```python
from build123d import *

# Parameters (mm, degrees)
F1_DEPTH = 5.842
F3_D     = 6.35
F4_SIZE  = 0.508


with BuildPart() as f1:
    # F0 (on Front) → F1 (new body)
    with BuildSketch(Plane.XZ):
        with BuildLine():
            ThreePointArc((-9.5238039492, 50.4641557941), (-0.0754731213, 40.7885133075), (9.525, 50.3132142901))
            ThreePointArc((9.525, 50.3132142901), (9.5247764361, 50.3784740944), (9.524105755, 50.4437308352))
            ThreePointArc((9.524105755, 50.4437308352), (0.0102135943, 59.8382088142), (-9.5238039492, 50.4641557941))
        make_face()
        with BuildLine():
            ThreePointArc((9.524105755, 50.4437308352), (9.5247764361, 50.3784740944), (9.525, 50.3132142901))
            ThreePointArc((9.525, 50.3132142901), (-0.0754731213, 40.7885133075), (-9.5238039492, 50.4641557941))
            Line((-9.5238039492, 50.4641557941), (-15.7481848278, 1.515787542))
            ThreePointArc((-15.7481848278, 1.515787542), (-0.7382390734, 15.3710397423), (15.4940214613, 2.9702251313))
            Line((15.4940214613, 2.9702251313), (9.524105755, 50.4437308352))
        make_face()
        with BuildLine():
            Line((15.8675349274, 0), (15.4940214613, 2.9702251313))
            ThreePointArc((15.4940214613, 2.9702251313), (-0.7382390734, 15.3710397423), (-15.7481848278, 1.515787542))
            ThreePointArc((-15.7481848278, 1.515787542), (-15.8446680698, 0.4940908149), (-15.8749364489, -0.5317049948))
            Line((-15.8749364489, -0.5317049948), (-15.404151012, -4.3244616471))
            ThreePointArc((-15.404151012, -4.3244616471), (-0.1436036046, -16.3611361849), (15.332202426, -4.602510891))
            Line((15.332202426, -4.602510891), (15.8675349274, 0))
        make_face()
        with BuildLine():
            ThreePointArc((15.8675349274, 0), (15.7509480386, 1.4939366044), (15.4940214613, 2.9702251313))
            Line((15.4940214613, 2.9702251313), (15.8675349274, 0))
        make_face()
        with BuildLine():
            ThreePointArc((-15.8749364489, -0.5317049948), (-15.8446680698, 0.4940908149), (-15.7481848278, 1.515787542))
            Line((-15.7481848278, 1.515787542), (-15.9409356657, 0))
            Line((-15.9409356657, 0), (-15.8749364489, -0.5317049948))
        make_face()
        with BuildLine():
            ThreePointArc((15.875, -0.4867857099), (15.8731336221, -0.2433642366), (15.8675349274, 0))
            Line((15.8675349274, 0), (15.332202426, -4.602510891))
            ThreePointArc((15.332202426, -4.602510891), (15.7387156165, -2.5624677046), (15.875, -0.4867857099))
        make_face()
        with BuildLine():
            Line((-15.404151012, -4.3244616471), (-15.8749364489, -0.5317049948))
            ThreePointArc((-15.8749364489, -0.5317049948), (-15.7540972084, -2.4423025589), (-15.404151012, -4.3244616471))
        make_face()
        with BuildLine():
            Line((10.9490243725, -42.2867999584), (15.332202426, -4.602510891))
            ThreePointArc((15.332202426, -4.602510891), (-0.1436036046, -16.3611361849), (-15.404151012, -4.3244616471))
            Line((-15.404151012, -4.3244616471), (-7.8770486042, -64.9645441344))
            ThreePointArc((-7.8770486042, -64.9645441344), (-0.4898126958, -56.0644129735), (7.9375, -63.9867857099))
            ThreePointArc((7.9375, -63.9867857099), (5.6126600757, -69.5994457855), (0, -71.9242857099))
            Line((0, -71.9242857099), (44.45, -71.9242857099))
            ThreePointArc((44.45, -71.9242857099), (36.5125, -63.9867857099), (44.45, -56.0492857099))
            Line((44.45, -56.0492857099), (17.3799107009, -51.0071446685))
            ThreePointArc((17.3799107009, -51.0071446685), (12.4451190536, -47.9149192836), (10.9490243725, -42.2867999584))
        make_face()
        with BuildLine():
            ThreePointArc((7.9375, -63.9867857099), (-0.4898126958, -56.0644129735), (-7.8770486042, -64.9645441344))
            ThreePointArc((-7.8770486042, -64.9645441344), (-5.2556136062, -69.9350990735), (0, -71.9242857099))
            ThreePointArc((0, -71.9242857099), (5.6126600757, -69.5994457855), (7.9375, -63.9867857099))
        make_face()
        with BuildLine():
            ThreePointArc((52.3875, -63.9867857099), (50.0626600757, -58.3741256342), (44.45, -56.0492857099))
            ThreePointArc((44.45, -56.0492857099), (36.5125, -63.9867857099), (44.45, -71.9242857099))
            ThreePointArc((44.45, -71.9242857099), (50.0626600757, -69.5994457855), (52.3875, -63.9867857099))
        make_face()
    extrude(amount=F1_DEPTH)

    # F3 (through all)
    with Locations(Plane(origin=(0, 0, 0), x_dir=(-1, 0, 0), z_dir=(0, 1, 0))):
        with Locations((0, 0)):
            Hole(F3_D / 2)

    # F4
    f4_edges = [f1.edges().sort_by_distance(p)[0] for p in [
        (-12.73237, 0, 25.232078),
    ]]
    chamfer(f4_edges, length=F4_SIZE)


solid = f1.part
```
Source: CAD feature listing. Evaluate the final solid. Frame: model axes, mm. A direction names the side the tool comes from. Round coordinates to 2 decimals unless told otherwise and drop trailing zeros. Loops run counter-clockwise (first coordinate to the right, second up) from the corner with the lowest first, then second, coordinate; pieces in that order, holes last.
(1) Section query D-D (z = -30.5). Output: boundary loops of the cut face in (x, y).
From the geometry:
outline: (-12.16, -5.84) - (12.32, -5.84) - (12.32, 0) - (-12.16, 0) - close
(2) Contact query for flat-ended pins moving along their axis: pin 1 Ø4 at (x, z) = (0, 0) entering from +Y; pin 2 Ø1 at (y, z) = (-3, 12.5) entering from -X (3 decimals); pin 3 Ø1.5 at (y, z) = (-4.5, -37.5) entering from +X; pin 4 Ø3 at (y, z) = (-4, -47.5) entering from -X. Output: stop coordinate, or through.
From the geometry:
pin 1: passes through
pin 2: stops at x = -14.415
pin 3: stops at x = 11.59
pin 4: stops at x = -10.23
(3) Material intervals for probe 1 along Z at (x, y) = (32, -0.25); probe 2 along X at (y, z) = (-0.35, -11); probe 3 along X at (y, z) = (-1.85, -58.5), sorted ascending.
From the geometry:
probe 1: z = -71.92 to -53.73
probe 2: x = -14.58 to 14.59
probe 3: x = -8.68 to 50.19
(4) Section query C-C (x = 47.5). Output: boundary loops of the cut face in (y, z), and give its area (3 significant figures).
From the geometry:
outline: (-5.84, -71.31) - (0, -71.31) - (0, -56.66) - (-5.84, -56.66) - close
area: 85.6 mm2
(5) Section query B-B (z = 31.5). Output: boundary loops of the cut face in (x, y).
From the geometry:
outline: (-11.94, -5.84) - (11.91, -5.84) - (11.91, 0) - (-11.42, 0) - (-11.94, -0.51) - close
(6) Pull-direction query (X, two-part tool) for faces 3 (the cylindrical face through (-0.69, -2.96, -3.1)), 4 (the cylindrical face through (-5.32, -2.88, -69.88)), 5 (the flat face through (3, -5.842, -20)), 6 (the flat face through (31.104, -2.88, -53.564)); classes: +X half, -X half, draft (parallel to the pull), parting line (faces both ways), or undercut.
From the geometry:
face 3: undercut
face 4: -X half
face 5: draft
face 6: +X half
(7) Access query for faces 1 (the flat face through (13.11, -2.88, -23.71)), 2 (the flat face through (22, -3, -71.924)). Directions: +Z, -Z, +X, -X, +Y, -Y. A direction counts if a zero-diameter tool reaches every point of the face in a straight line with its end or side. Return the directions, or none.
From the geometry:
face 1: +X, +Y, -Y
face 2: -Z, +X, -X, +Y, -Y
